The listing builds one solid part. Answer for the finished solid, in the listing's coordinates (mm). Face numbers are marked on the shaded views. Coordinates: 2 decimals unless noted, no trailing zeros. Write each loop counter-clockwise with the first axis right and the second up, starting at its lowest first coordinate (ties: lowest second). Pieces come first, ordered by that corner, then holes.
(1) The part is cut by section A-A on z = 7. Determine the outline of the cut face in (x, y), plus the area to 3 significant figures.
(2) Straight lines are drawn through the part: line 1 (Y direction, x = -4.5, z = 7.5); line 2 (X direction, y = -43, z = 2); line 3 (Z direction, x = -7.5, y = -64). For each, find the intervals that lie inside material, in ascending order.
(3) The part is cut by section C-C on x = -20.5. Determine the outline of the cut face in (y, z).
(4) Given P1, Ø1, axis at y = -77, z = 11.5, coming from the -X side; P2, Ø7.5, axis at x = -32.64, y = -43.22, coming from the -Z side; P3, Ø12, axis at x = -21, y = -75, coming from the -Z side; P4, Ø3.5, axis at x = -53.38, y = -75.18, coming from the -Z side, each flat-ended and moving along its own axis, determine where each tip first touches the part or whether it passes through.
(5) For a pull along Z with two mould halves and no side action, classify the marked faces 1, 2 and 3 as +Z half, -Z half, draft (parallel to the pull), parting line (faces both ways), or undercut.
(6) The part is cut by section B-B on y = -47.5. Determine the outline of the cut face in (x, z).
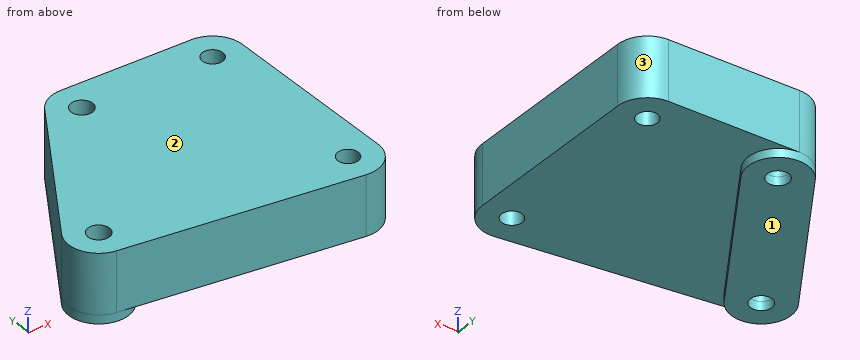
Autodesk Inventor part; units mm, degrees
ref_plane "Work Plane2" through (-11.9062, -368.3, 1.8415) normal (0, 0, 1) x (1, 0, 0)
ref_plane "YZ Plane" through (0, 0, 0) normal (1, 0, 0) x (0, 1, 0)
ref_plane "XZ Plane" through (0, 0, 0) normal (0, 1, 0) x (-1, 0, 0)
ref_plane "Work Plane1" through (0, 0, 0) normal (0, 0, 1) x (1, 0, 0)
sketch "Sketch1" plane through (0, 0, 0) normal (0, 0, 1) x (1, 0, 0)
  circle A0 centre (-53.3761, -75.183) radius 2.286
  circle A1 centre (-32.6369, -43.2221) radius 2.286
  line L0 (-53.3761, -75.183) -> (-32.6369, -43.2221) construction
  line L1 (-48.0493, -78.6395) -> (-27.3101, -46.6786)
  line L2 (-37.9638, -39.7656) -> (-58.7029, -71.7265)
  arc A2 (-58.7029, -71.7265) -> (-48.0493, -78.6395) centre (-53.3761, -75.183) ccw
  arc A3 (-27.3101, -46.6786) -> (-37.9638, -39.7656) centre (-32.6369, -43.2221) ccw
  line L3 (-55.5272, -90.1636) -> (-13.3531, -25.1695)
  point P0 (0, 0)
  point P1 (-43.0065, -59.2025)
ref_plane "Work Plane2" through (-11.9062, -368.3, 1.8415) normal (0, 0, 1) x (1, 0, 0)
extrude "Extrusion1" add sketch "Sketch1" along normal up to surface (1.8415 mm away)
sketch "Sketch2" plane through (-58.7029, -71.7265, 1.8415) normal (0, 0, 1) x (0.8388686, -0.544334, 0)
  circle A0 centre (29.7355, 51.8109) radius 2.1844
  circle A1 centre (50.4747, 19.85) radius 2.1844
  line L0 (0, 0) -> (0, 38.1)
  arc A2 (0, 0) -> (12.7, 0) centre (6.35, 0) ccw
  line L1 (12.7, 38.1) -> (12.7, 0)
  arc A3 (12.7, 38.1) -> (0, 38.1) centre (6.35, 38.1) ccw
  circle A4 centre (6.35, 0) radius 2.286
  circle A5 centre (6.35, 38.1) radius 2.286
  arc A6 (35.0623, 55.2674) -> (26.5238, 57.2888) centre (29.7355, 51.8109) ccw
  arc A7 (53.0798, 14.059) -> (55.8015, 23.3065) centre (50.4747, 19.85) ccw
  line L2 (26.5238, 57.2888) -> (3.1383, 43.5779)
  line L3 (35.0623, 55.2674) -> (55.8015, 23.3065)
  line L4 (53.0798, 14.059) -> (8.9552, -5.791)
  point P0 (10.2009, 92.1231)
  dimension "d2" = 12.7
  dimension "d3" = 12.7
extrude "Extrusion2" add sketch "Sketch2" along normal blind 12.7
properties part number "Intake"
Model answer:
1. outline: (-58.7, -71.73) arc R6.35 ccw to (-54.34, -81.46) - (-6.52, -88.83) arc R6.35 ccw to (0.79, -82.55) - (0.79, -44.45) arc R6.35 ccw to (-5.27, -38.11) - (-32.35, -36.88) arc R6.35 ccw to (-37.96, -39.77) - close; hole circle Ø4.57 at (-53.38, -75.18); hole circle Ø4.57 at (-32.64, -43.22); hole circle Ø4.37 at (-5.56, -82.55); hole circle Ø4.37 at (-5.56, -44.45)
1. area: 2,380 mm2
2. line 1: y = -88.81 to -84.46, -80.64 to -46.36, -42.54 to -38.19
2. line 2: x = -40.06 to -34.91, -30.36 to -7.19, -3.92 to 0.63
2. line 3: z = 1.84 to 14.54
3. outline: (-86.67, 1.84) - (-37.42, 1.84) - (-37.42, 14.54) - (-86.67, 14.54) - close
4. P1: stops at x = -59.59
4. P2: stops at z = 0
4. P3: stops at z = 1.84
4. P4: passes through
5. face 1: -Z half
5. face 2: +Z half
5. face 3: draft
6. outline: (-42.98, 0) - (-27.84, 0) - (-27.84, 1.84) - (0.79, 1.84) - (0.79, 14.54) - (-42.98, 14.54) - close
